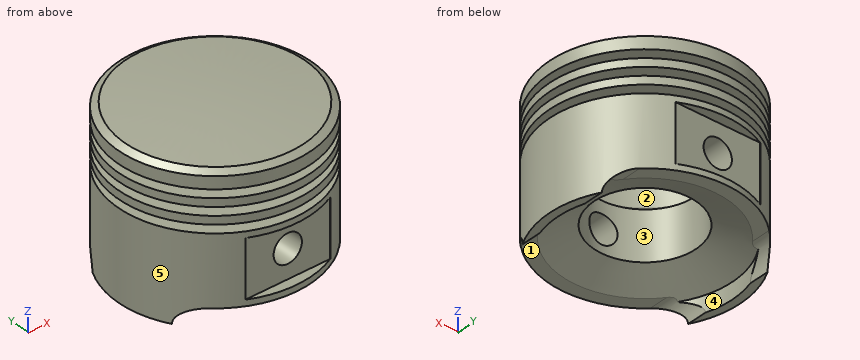
from build123d import *

# Parameters (mm, degrees)
F2_R     = 7
F3_DEPTH = 72
F5_START = 42
F4_W     = 42
F4_H     = 28
F4_R     = 7
F5_DEPTH = 28.7
F9_DEPTH = 211.3


# Not quite as in the source:
# - a pattern or mirror of a feature is missing from the dataset's text; its kind, count and spacing are read off the source's solid


with BuildPart() as f1:
    # F0 (on Front) → F1 (revolve)
    with BuildSketch(Plane.XZ):
        with BuildLine():
            Line((47, 87), (43.7432713807, 89))
            ThreePointArc((43.7432713807, 89), (21.8944844144, 90.4997389679), (0, 91))
            Line((0, 91), (0, 18))
            Line((0, 18), (47, 18))
            Line((47, 18), (47, 33))
            Line((47, 33), (47, 57))
            Line((47, 57), (47, 61))
            Line((47, 61), (41, 61))
            Line((41, 61), (41, 65))
            Line((41, 65), (47, 65))
            Line((47, 65), (47, 69))
            Line((47, 69), (41, 69))
            Line((41, 69), (41, 73))
            Line((41, 73), (47, 73))
            Line((47, 73), (47, 77))
            Line((47, 77), (41, 77))
            Line((41, 77), (41, 81))
            Line((41, 81), (47, 81))
            Line((47, 81), (47, 87))
        make_face()
    revolve(axis=Axis((0, 0, 45.5), (0, 0, -1)))

    # F2 (on Front) → F3 (cut, symmetric)
    with BuildSketch(Plane.XZ):
        with Locations((0, 44)):
            Circle(F2_R)
    extrude(amount=F3_DEPTH, both=True, mode=Mode.SUBTRACT)

    # F4 (on Front) → F5 (cut)
    with BuildSketch(Plane.XZ.offset(F5_START)):
        with Locations((0, 44)):
            Rectangle(F4_W, F4_H)
        with Locations((0, 44)):
            Circle(F4_R, mode=Mode.SUBTRACT)
    f5 = extrude(amount=F5_DEPTH, mode=Mode.SUBTRACT)

    # F5_copies: F5 across plane
    add(f5.mirror(Plane.ZX), mode=Mode.SUBTRACT)

    # F6 (on Front) → F7 (revolve, cut)
    with BuildSketch(Plane.XZ):
        with BuildLine():
            Line((0, 81), (0, 18))
            Line((0, 18), (43, 18))
            Line((43, 18), (43, 26))
            Line((43, 26), (25, 33))
            Line((25, 33), (25, 57))
            Line((25, 57), (28, 57))
            ThreePointArc((28, 57), (33.6568542495, 59.3431457505), (36, 65))
            Line((36, 65), (36, 81))
            Line((36, 81), (0, 81))
        make_face()
    revolve(axis=Axis((0, 0, 34.176344052), (0, 0, 1)), mode=Mode.SUBTRACT)

    # F8 (on Front) → F9 (cut, symmetric)
    with BuildSketch(Plane.XZ):
        with BuildLine():
            Line((32, 27), (-32, 27))
            ThreePointArc((-32, 27), (-38.3639610307, 24.3639610307), (-41, 18))
            Line((-41, 18), (41, 18))
            ThreePointArc((41, 18), (38.3639610307, 24.3639610307), (32, 27))
        make_face()
    extrude(amount=F9_DEPTH, both=True, mode=Mode.SUBTRACT)


solid = f1.part
Verification items for the finished model (mm, model axes). Face numbers are marked on the shaded views. A direction names the side the tool comes from. Round coordinates to 2 decimals unless told otherwise and drop trailing zeros. Order: outer loops, then holes, each group sorted by start corner. A loop starts at its lowest first (then second) coordinate and runs counter-clockwise, first axis right, second up.
1. Go/stop test with flat-tipped pins: P1, Ø12, axis at y = 26, z = 55.5, coming from the -X side; P2, Ø12, axis at x = -30.5, y = -13, coming from the +Z side; P3, Ø2, axis at y = 3.5, z = 61, coming from the -X side. Record where each tip stops, or that it passes through.
Final values:
P1: stops at x = -42.53
P2: stops at z = 90.23
P3: stops at x = -46.93
2. Thickness scan on L1, parallel to Y at x = 0, z = 71; L2, parallel to Z at x = 0, y = 30; L3, parallel to Z at x = -6.5, y = -42.5. Record the ranges inside material, lowest first.
Final values:
L1: y = -41 to -36, 36 to 41
L2: z = 31.06 to 37, 51 to 57.25, 81 to 90.06
L3: z = 27 to 30, 58 to 61, 65 to 69, 73 to 77, 81 to 89.07
3. Access from +Z, -Z, +X, -X, +Y, -Y to the whole of each face (thin tool, end or side, straight path). Record for the marked faces 1, 2 and 3.
Final values:
face 1: -Z, +Y, -Y
face 2: none
face 3: -Z
4. Section check B-B on z = 55. Record the cut outline in (x, y), then the cut area to 3 significant figures.
Final values:
outline: (-21, -42.05) - (-21, -42) - (21, -42) - (21, -42.05) arc R47 ccw to (21, 42.05) - (21, 42) - (-21, 42) - (-21, 42.05) arc R47 ccw to start; hole circle Ø50 at (0, 0)
area: 4,690 mm2
5. Section check C-C on x = 0. State how many separate pieces and enclosed holes the cut face has, then the cut area to 3 significant figures.
Final values:
separate pieces: 3
enclosed holes: 0
area: 1,750 mm2
6. Section check A-A on z = 44. Record the cut outline in (x, y), then the cut area to 3 significant figures.
Final values:
outline: (-21, -42.05) - (-21, -42) - (-7, -42) - (-7, -24) arc R25 cw to (-7, 24) - (-7, 42) - (-21, 42) - (-21, 42.05) arc R47 ccw to start; (7, -42) - (21, -42) - (21, -42.05) arc R47 ccw to (21, 42.05) - (21, 42) - (7, 42) - (7, 24) arc R25 cw to (7, -24) - close
area: 4,210 mm2
7. Release check for a two-part mould opening along X. For the marked faces 4 and 5 record: +X half, -X half, draft (parallel to the pull), parting line (faces both ways), or undercut.
Final values:
face 4: undercut
face 5: parting line
8. Section check D-D on z = 82.5. Record the cut outline in (x, y).
Final values:
outline: circle Ø94 at (0, 0)
